from build123d import *

# Parameters (mm, degrees)
SKETCH_1_W      = 13.5
SKETCH_1_H      = 18
EXTRUDE_1_DEPTH = 1
SKETCH_2_W      = 3
SKETCH_2_H      = 5
EXTRUDE_2_DEPTH = 0.2
SKETCH_3_W      = 5
SKETCH_3_H      = 5
EXTRUDE_3_DEPTH = 2


with BuildPart() as part:
    # Эскиз1 → Бобышка-Вытянуть1 (new body)
    with BuildSketch(Plane(origin=(0, 0, 0), x_dir=(1, 0, 0), z_dir=(0, 1, 0))):
        Rectangle(SKETCH_1_W, SKETCH_1_H)
    extrude(amount=EXTRUDE_1_DEPTH)

    # Эскиз2 → Бобышка-Вытянуть2 (add)
    with BuildSketch(Plane(origin=(0, 1, 0), x_dir=(1, 0, 0), z_dir=(0, 1, 0))):
        with Locations((-5.25, -6.5)):
            Rectangle(SKETCH_2_W, SKETCH_2_H)
        with Locations((5.25, -6.5)):
            Rectangle(SKETCH_2_W, SKETCH_2_H)
        with Locations((-5.25, 6.5)):
            Rectangle(SKETCH_2_W, SKETCH_2_H)
        with Locations((5.25, 6.5)):
            Rectangle(SKETCH_2_W, SKETCH_2_H)
    extrude(amount=EXTRUDE_2_DEPTH)

    # Эскиз3 → Бобышка-Вытянуть3 (add)
    with BuildSketch(Plane(origin=(0, 1, 0), x_dir=(1, 0, 0), z_dir=(0, 1, 0))):
        with Locations((3.75, 0)):
            Rectangle(SKETCH_3_W, SKETCH_3_H)
    extrude(amount=EXTRUDE_3_DEPTH)


solid = part.part
Build history of the part. All positions in model axes, mm. A direction names the side the tool comes from. Round coordinates to 2 decimals unless told otherwise and drop trailing zeros. Order: outer loops, then holes, each group sorted by start corner. A loop starts at its lowest first (then second) coordinate and runs counter-clockwise, first axis right, second up. Notation, with made-up numbers: M -30.5,73 L -21.5,73 A19 cw -21.5,99 Z; hole C -11.5,49 d5. An arc over 180 degrees is marked long. Use CSV: the item, a comma, the result in double quotes. Start each with the question number.
(1) Tool access for faces 4 (the face through (-6.75, 0.6, 0.1)), 5 (the face through (5, 1.2, -7)), 6 (the face through (6.75, 0.6, 0.1)), 7 (the face through (5, 1.2, 6)), 8 (the face through (1.25, 2, 0)): list every direction of +Z, -Z, +X, -X, +Y, -Y with a clear straight run to the whole face (end or side of a thin tool).
(2) Cut at B-B on z = -1. List the corners of the cut face in (x, y).
(3) Cut at A-A on x = 4.25. List the corners of the cut face in (y, z).
(4) Cut at D-D on z = 4.5. List the corners of the cut face in (x, y), then the cut area to 3 significant figures.
(5) Cut at C-C on y = 1.8. List the corners of the cut face in (x, z).
(6) Mould opens along Z. For faces 1 (the face through (-2, 1, 0)), 2 (the face through (-5, 1.2, -7)), 3 (the face through (-0.1, 0.6, 9)) say: +Z half, -Z half, draft (parallel to the pull), parting line (faces both ways), or undercut.
(7) Drill centre lines: probe 1 along Y at (x, z) = (-2.25, -0.25); probe 2 along X at (y, z) = (2.55, -0.5); probe 3 along Z at (x, y) = (5.5, 2.65). Where is each one in solid material? Low to high.
(8) Flat gauge pins, fed straight in: P1, Ø1.6, axis at x = 4, y = 2.5, coming from the +Z side; P2, Ø1.5, axis at x = 6, z = -7.5, coming from the +Y side; P3, Ø6, axis at x = -1.5, z = 3, coming from the -Y side; P4, Ø1, axis at y = 2, z = -0.5, coming from the -X side. Where does each tip first touch, or does it go through?
Findings:
1,face 4,"+Z, -Z, -X, +Y, -Y"
1,face 5,"-Z, +X, -X, +Y"
1,face 6,"+Z, -Z, +X, +Y, -Y"
1,face 7,"+Z, +X, -X, +Y"
1,face 8,"+Z, -Z, -X, +Y"
2,outline,"M -6.75,0 L 6.75,0 L 6.75,1 L 6.25,1 L 6.25,3 L 1.25,3 L 1.25,1 L -6.75,1 Z"
3,outline,"M 0,-9 L 1.2,-9 L 1.2,-4 L 1,-4 L 1,-2.5 L 3,-2.5 L 3,2.5 L 1,2.5 L 1,4 L 1.2,4 L 1.2,9 L 0,9 Z"
4,outline,"M -6.75,0 L 6.75,0 L 6.75,1.2 L 3.75,1.2 L 3.75,1 L -3.75,1 L -3.75,1.2 L -6.75,1.2 Z"
4,area,"14.7 mm^2"
5,outline,"M 1.25,-2.5 L 6.25,-2.5 L 6.25,2.5 L 1.25,2.5 Z"
6,face 1,"undercut"
6,face 2,"draft"
6,face 3,"+Z half"
7,probe 1,"y = 0 to 1"
7,probe 2,"x = 1.25 to 6.25"
7,probe 3,"z = -2.5 to 2.5"
8,P1,"stops at z = 2.5"
8,P2,"stops at y = 1.2"
8,P3,"stops at y = 0"
8,P4,"stops at x = 1.25"
